Autodesk Inventor part; units mm, degrees
ref_plane "YZ Plane" through (0, 0, 0) normal (1, 0, 0) x (0, 1, 0)
ref_plane "XZ Plane" through (0, 0, 0) normal (0, 1, 0) x (-1, 0, 0)
ref_plane "XY Plane" through (0, 0, 0) normal (0, 0, 1) x (1, 0, 0)
sketch "Sketch1" plane through (0, 0, 0) normal (0, 0, 1) x (1, 0, 0)
  line L0 (0, 0) -> (30, 0)
  line L1 (30, 0) -> (30, 4)
  line L2 (30, 4) -> (68, 4)
  line L3 (68, 4) -> (68, 20)
  line L4 (68, 20) -> (24, 20)
  line L5 (24, 20) -> (24, 16)
  line L6 (24, 16) -> (0, 16)
  line L7 (0, 16) -> (0, 0)
  dimension "d0" = 30
  dimension "d1" = 4
  dimension "d2" = 38
  dimension "d3" = 16
  dimension "d4" = 44
  dimension "d5" = 4
extrude "Extrusion1" add sketch "Sketch1" against normal blind 82
sketch "Sketch2" plane through (24, 20, 0) normal (0, 1, 0) x (1, 0, 0)
  circle A0 centre (32, 12) radius 5.5
  circle A1 centre (32, 70) radius 5.5
  line L0 (44, 0) -> (44, 82)
  line L1 (44, 0) -> (0, 0)
  line L2 (0, 82) -> (44, 82)
  point P0 (-24, 0)
  dimension "d8" = 11
  dimension "d9" = 11
  dimension "d10" = 12
  dimension "d11" = 12
  dimension "d12" = 12
  dimension "d13" = 12
extrude "Extrusion2" cut sketch "Sketch2" against normal blind 82 contours A0
extrude "Extrusion3" cut sketch "Sketch2" against normal blind 82 contours A1
fillet "Fillet1" radius 12 1 edges at (68, 12, 0)
fillet "Fillet2" radius 12 1 edges at (68, 12, -82)
mirror "Mirror1" about plane through (0, 0, 0) normal (1, 0, 0) of "Extrusion1", "Fillet1", "Extrusion2", "Extrusion3", "Fillet2"
properties part number "topPlate" material "Steel, Carbon"
For this review, take the finished solid that the model builds, in its own axes (mm). A direction names the side the tool comes from. Give positions to 0.01 mm unless a question says otherwise; leave off trailing zeros. Order: outer loops, then holes, each group sorted by start corner. A loop starts at its lowest first (then second) coordinate and runs counter-clockwise, first axis right, second up. Notation, with made-up numbers: M 39,9.25 L 72,9.25 A21 ccw 72,35.25 Z; hole C -1,-34.5 d1. An arc over 180 degrees is marked long. Answer in a Markdown table with one row per item. Add a question column.
(1) Wall thickness on probe 1 along Z at (x, y) = (56, 11); probe 2 along X at (y, z) = (15.5, -70); probe 3 along X at (y, z) = (19, -20): over which ranges is each line inside the solid? List them lowest first. Write a range as [from, to].
(2) For faces 1 (the face through (-64.58, 12.11, -3.61)), 2 (the face through (30, 2, -40)), 3 (the face through (24, 18, -40)), 4 (the face through (-49, 4, -40)), 5 (the face through (-1, 10, -82)), list the 3-axis set-ups (+Z, -Z, +X, -X, +Y, -Y) from which the entire face can be reached by the end or side of a thin tool; tool diameter is ignored.
(3) For pin 1 (10 mm diameter, centred on x = -56, z = -70, fed in from +Y); pin 2 (12.5 mm diameter, centred on x = 56, z = -70, fed in from -Y); pin 3 (6 mm diameter, centred on y = 3.5, z = -73.5, fed in from +X); pin 4 (14.5 mm diameter, centred on x = -11, z = -41, fed in from +Y), all flat-tipped, find the tip position at first contact; note any pin that passes through.
(4) Mouldability with a two-part tool opening along X and no side actions: class faces 6 (the face through (64.58, 12.11, -78.39)), 7 (the face through (50.505, 12.112, -12.242)), 8 (the face through (-68, 12, -41)) as +X half, -X half, draft (parallel to the pull), parting line (faces both ways), or undercut.
(5) Consider section A-A on z = -25.5. State the section outline as (x, y) points, and give its area (3 significant figures).
(6) Consider section C-C on x = 36. State the section outline as (y, z) points, and give its area (3 significant figures).
(7) Consider section B-B on y = 11.75. State the section outline as (x, z) points.
Evaluation:
| question | item | result |
|---|---|---|
| 1 | probe 1 | z = [-82, -75.5], [-64.5, -17.5], [-6.5, 0] |
| 1 | probe 2 | x = [-68, -61.5], [-50.5, 50.5], [61.5, 68] |
| 1 | probe 3 | x = [-68, -24], [24, 68] |
| 2 | face 1 | +Z, -X, +Y, -Y |
| 2 | face 2 | +Z, -Z, +X, -Y |
| 2 | face 3 | +Z, -Z, +Y |
| 2 | face 4 | +Z, -Z, -X, -Y |
| 2 | face 5 | -Z, +X, -X, +Y, -Y |
| 3 | pin 1 | passes through |
| 3 | pin 2 | stops at y = 4 |
| 3 | pin 3 | stops at x = 67.99 |
| 3 | pin 4 | stops at y = 16 |
| 4 | face 6 | +X half |
| 4 | face 7 | undercut |
| 4 | face 8 | -X half |
| 5 | outline | M -68,4 L -30,4 L -30,0 L 30,0 L 30,4 L 68,4 L 68,20 L 24,20 L 24,16 L -24,16 L -24,20 L -68,20 Z |
| 5 | area | 2,220 mm^2 |
| 6 | outline | M 4,-82 L 20,-82 L 20,0 L 4,0 Z |
| 6 | area | 1,310 mm^2 |
| 7 | outline | M -68,-70 A12 ccw -56,-82 L 56,-82 A12 ccw 68,-70 L 68,-12 A12 ccw 56,0 L -56,0 A12 ccw -68,-12 Z; hole C -56,-70 d11; hole C -56,-12 d11; hole C 56,-70 d11; hole C 56,-12 d11 |
